from build123d import *

# Parameters (mm, degrees)
BOSS_EXTRUDE1_DEPTH = 20
SKETCH2_R           = 2.1
CUT_EXTRUDE1_DEPTH  = 20
SKETCH3_R           = 2.098017688
SKETCH3_R_2         = 2.10074066
CUT_EXTRUDE2_DEPTH  = 20
SKETCH7_R           = 6
BOSS_EXTRUDE2_DEPTH = 1.5
SKETCH8_R           = 4.804871241
BOSS_EXTRUDE3_DEPTH = 0.5
SKETCH9_R           = 4.002646766
CUT_EXTRUDE5_DEPTH  = 2.5
SKETCH10_OUTSIDE_W  = 68.236
SKETCH10_OUTSIDE_H  = 35.636
CUT_EXTRUDE6_DEPTH  = 2.5
BOSS_EXTRUDE4_DEPTH = 2.5


with BuildPart() as part:
    # Sketch1 → Boss-Extrude1 (new body)
    with BuildSketch(Plane.XY):
        with BuildLine():
            Line((-2, 0), (-38, 0))
            ThreePointArc((-38, 0), (-39.414213562, 0.585786438), (-40, 2))
            Line((-40, 2), (-40, 26.5))
            Line((-40, 26.5), (-46.3, 26.5))
            Line((-46.3, 26.5), (-46.3, 29.5))
            Line((-46.3, 29.5), (-40, 29.5))
            Line((-40, 29.5), (-40, 34))
            Line((-40, 34), (-33, 34))
            Line((-33, 34), (-33, 36.5))
            Line((-33, 36.5), (0, 36.5))
            Line((0, 36.5), (0, 29.5))
            Line((0, 29.5), (6.3, 29.5))
            Line((6.3, 29.5), (6.3, 26.5))
            Line((6.3, 26.5), (0, 26.5))
            Line((0, 26.5), (0, 2))
            ThreePointArc((0, 2), (-0.585786438, 0.585786438), (-2, 0))
        make_face()
    extrude(amount=BOSS_EXTRUDE1_DEPTH)

    # Sketch2 → Cut-Extrude1 (cut)
    with BuildSketch(Plane(origin=(0, 29.5, 0), x_dir=(1, 0, 0), z_dir=(0, 1, 0))):
        with Locations(Location((3.8, -15.10338686, 0), (0, 0, 270))):
            Circle(SKETCH2_R)
        with Locations(Location((3.8, -4.896599974, 0), (0, 0, 270))):
            Circle(SKETCH2_R)
    extrude(amount=-CUT_EXTRUDE1_DEPTH, mode=Mode.SUBTRACT)

    # Sketch3 → Cut-Extrude2 (cut)
    with BuildSketch(Plane(origin=(0, 29.5, 0), x_dir=(1, 0, 0), z_dir=(0, 1, 0))):
        with Locations(Location((-43.799859357, -15.098694551, 0), (0, 0, 270))):
            Circle(SKETCH3_R)
        with Locations(Location((-43.799859357, -4.903327435, 0), (0, 0, 270))):
            Circle(SKETCH3_R_2)
    extrude(amount=-CUT_EXTRUDE2_DEPTH, mode=Mode.SUBTRACT)

    # Sketch7 → Boss-Extrude2 (add)
    with BuildSketch(Plane(origin=(0, 36.5, 0), x_dir=(1, 0, 0), z_dir=(0, 1, 0))):
        with Locations(Location((-10.95500567, -10, 0), (0, 0, 90))):
            Circle(SKETCH7_R)
    extrude(amount=BOSS_EXTRUDE2_DEPTH)

    # Sketch8 → Boss-Extrude3 (add)
    with BuildSketch(Plane(origin=(0, 38, 0), x_dir=(1, 0, 0), z_dir=(0, 1, 0))):
        with Locations(Location((-10.95500567, -10, 0), (0, 0, 270))):
            Circle(SKETCH8_R)
    extrude(amount=BOSS_EXTRUDE3_DEPTH)

    # Sketch9 → Cut-Extrude5 (cut)
    with BuildSketch(Plane(origin=(0, 38.5, 0), x_dir=(1, 0, 0), z_dir=(0, 1, 0))):
        with Locations(Location((-10.95500567, -10, 0), (0, 0, 270))):
            Circle(SKETCH9_R)
    extrude(amount=-CUT_EXTRUDE5_DEPTH, mode=Mode.SUBTRACT)

    # Sketch10 outside → Cut-Extrude6 (cut)
    with BuildSketch(Plane(origin=(0, 36.5, 0), x_dir=(1, 0, 0), z_dir=(0, 1, 0))):
        with Locations((-20, -10)):
            Rectangle(SKETCH10_OUTSIDE_W, SKETCH10_OUTSIDE_H)
        with BuildLine():
            Line((-32.027169465, -18.996750159), (-10.95500567, -18.996750159))
            ThreePointArc((-10.95500567, -18.996750159), (-1.954759683, -9.996504172), (-10.95500567, -0.996258185))
            Line((-10.95500567, -0.996258185), (-32.027169465, -0.996258185))
            Line((-32.027169465, -0.996258185), (-32.027169465, -18.996750159))
        make_face(mode=Mode.SUBTRACT)
    extrude(amount=-CUT_EXTRUDE6_DEPTH, mode=Mode.SUBTRACT)

    # Sketch11 → Boss-Extrude4 (add)
    with BuildSketch(Plane(origin=(0, 36.5, 0), x_dir=(1, 0, 0), z_dir=(0, 1, 0))):
        with BuildLine():
            Line((-32.027169465, -12.502490339), (-32.027169465, -7.490518005))
            ThreePointArc((-32.027169465, -7.490518005), (-32.914070297, -8.60654479), (-33.230490565, -9.996504172))
            ThreePointArc((-33.230490565, -9.996504172), (-32.914070297, -11.386463554), (-32.027169465, -12.502490339))
        make_face()
    extrude(amount=-BOSS_EXTRUDE4_DEPTH)


solid = part.part
Geometry: final body of the model. Coordinates: model frame, mm. A direction names the side the tool comes from. Coordinates: 2 decimals unless noted, no trailing zeros. Loops run counter-clockwise (first coordinate to the right, second up) from the corner with the lowest first, then second, coordinate; pieces in that order, holes last. Notation, with made-up numbers: (52.25, 58) - (88.25, 58) arc R15 ccw to (88.25, 78) - close; hole circle Ø8 at (-19.5, 12.25). An arc over 180 degrees is marked (long way). Put each result on its own line as item: value. Start each with the question number.
Q1. Cut plane B-B, the plane x = -22. Return loops of the section in (y, z).
Q2. Pull-direction query (Z, two-part tool) for faces 6 (the flat face through (6.3, 28, 10)), 7 (the cylindrical face through (-45.664, 28.021, 5.873)), 8 (the cylindrical face through (-13.88, 38.25, 6.19)), 9 (the flat face through (-11, 36, 10)); classes: released by +Z, released by -Z, zero draft, split by the parting line, or undercut.
Q3. Pin query (flat end, axial travel): pin 1 Ø10 at (y, z) = (15.5, 6) entering from +X; pin 2 Ø4 at (x, z) = (3.8, 4.9) entering from +Y; pin 3 Ø5 at (x, z) = (3.8, 15.1) entering from -Y; pin 4 Ø0.8 at (y, z) = (35, 5) entering from -X. Return the tip coordinate at first contact, or that it passes through.
Q4. Cut plane D-D, the plane y = 4.5. Return loops of the section in (x, z), and give its area (3 significant figures).
Q5. Set-up query: faces 1 (the flat face through (-21, 35, 0.996)), 2 (the cylindrical face through (-13.391, 37.268, 6.824)), 3 (the flat face through (0, 14, 10)), 4 (the flat face through (-22, 35, 18.997)), 5 (the flat face through (3, 29.5, 10)). Return all of +Z, -Z, +X, -X, +Y, -Y with unobstructed straight access to the full face (end or side cutting, diameter ignored); none if empty.
Q6. Cut plane A-A, the plane x = 3.8. Return loops of the section in (y, z), and give its area (3 significant figures).
Q7. Line query: line 1 (Y direction, x = -26.5, z = 13.5); line 2 (X direction, y = 14.5, z = 7.75); line 3 (X direction, y = 37.7, z = 10) (3 decimals). Output: solid intervals per line, ascending.
Filled sheet:
1. outline: (0, 0) - (34, 0) - (34, 1) - (36.5, 1) - (36.5, 19) - (34, 19) - (34, 20) - (0, 20) - close
2. face 6: zero draft
2. face 7: undercut
2. face 8: split by the parting line
2. face 9: undercut
3. pin 1: x = 0
3. pin 2: through
3. pin 3: y = 26.5
3. pin 4: x = -32.03
4. outline: (-40, 0) - (0, 0) - (0, 20) - (-40, 20) - close
4. area: 800 mm²
5. face 1: -Z, +X, -X, +Y
5. face 2: +Y
5. face 3: +Z, -Z, +X, -Y
5. face 4: +Z, +X, -X, +Y
5. face 5: +Z, -Z, +X, +Y
6. outline: (26.5, 0) - (29.5, 0) - (29.5, 2.8) - (26.5, 2.8) - close; (26.5, 7) - (29.5, 7) - (29.5, 13) - (26.5, 13) - close; (26.5, 17.2) - (29.5, 17.2) - (29.5, 20) - (26.5, 20) - close
6. area: 34.8 mm²
7. line 1: 0 to 36.5
7. line 2: -40 to 0
7. line 3: -16.955 to -14.958, -6.952 to -4.955
